CAD build for the part. Positions are in the model's coordinates, mm. Round coordinates to 2 decimals unless told otherwise and drop trailing zeros. Write each loop counter-clockwise with the first axis right and the second up, starting at its lowest first coordinate (ties: lowest second). Pieces come first, ordered by that corner, then holes. Notation, with made-up numbers: (11, 62) -> (62, 62) arc R28 cw to (62, 84) -> close; hole circle Ø11 at (80, 35). An arc over 180 degrees is marked (long way). Put each result on its own line as item: value. Start each with the question number.
1. Saw through at B-B on z = 1.85. List the corners of the cut face in (x, y), and give its area (3 significant figures).
2. Drill centre lines: line 1 (Y direction, x = 54, z = 1.7); line 2 (Y direction, x = -5.5, z = 2); line 3 (X direction, y = 4.5, z = 1.25). Where is each one in solid material? Low to high. Write a range as from..to.
3. Pull direction Y, two halves, no side cores. Call faces 1 (the cylindrical face through (60.49, 12.15, 2.03)), 2 (the cylindrical face through (52.52, 8.61, 1.97)), 3 (the flat face through (-1, 0, 4)): pulls with the +Y half, pulls with the -Y half, needs draft (parallel to the pull), parting line crosses it, or undercut.
4. Flat gauge pins, fed straight in: P1, Ø2.5, axis at x = 54, y = -8, coming from the -Z side; P2, Ø1, axis at y = -6, z = 2.5, coming from the -X side. Where does each tip first touch, or does it go through?
5. Saw through at A-A on x = -13.5. List the corners of the cut face in (y, z).
from build123d import *

# Parameters (mm, degrees)
ESBO_O1_W                = 127
ESBO_O1_H                = 30
ESBO_O1_R                = 3
ESBO_O1_R_2              = 1.6
RESSALTO_EXTRUS_O1_DEPTH = 4
FILETE1_R                = 10


with BuildPart() as part:
    # Esboço1 → Ressalto-extrusão1 (new body)
    with BuildSketch(Plane.XY):
        Rectangle(ESBO_O1_W, ESBO_O1_H)
        with Locations((-13.5, 4)):
            Circle(ESBO_O1_R, mode=Mode.SUBTRACT)
        with Locations((-5.5, 4)):
            Circle(ESBO_O1_R_2, mode=Mode.SUBTRACT)
        with Locations((-21.5, 4)):
            Circle(ESBO_O1_R_2, mode=Mode.SUBTRACT)
        with Locations((-54, 8)):
            Circle(ESBO_O1_R_2, mode=Mode.SUBTRACT)
        with Locations(Location((-54, -8, 0), (0, 0, 180))):
            Circle(ESBO_O1_R_2, mode=Mode.SUBTRACT)
        with Locations((54, -8)):
            Circle(ESBO_O1_R_2, mode=Mode.SUBTRACT)
        with Locations(Location((54, 8, 0), (0, 0, 180))):
            Circle(ESBO_O1_R_2, mode=Mode.SUBTRACT)
    extrude(amount=RESSALTO_EXTRUS_O1_DEPTH)

    # Filete1
    filete1_edges = [part.edges().sort_by_distance(p)[0] for p in [
        (63.5, -15, 2),
        (-63.5, -15, 2),
        (-63.5, 15, 2),
        (63.5, 15, 2),
    ]]
    fillet(filete1_edges, radius=FILETE1_R)


solid = part.part
Return value:
1. outline: (-63.5, -5) arc R10 ccw to (-53.5, -15) -> (53.5, -15) arc R10 ccw to (63.5, -5) -> (63.5, 5) arc R10 ccw to (53.5, 15) -> (-53.5, 15) arc R10 ccw to (-63.5, 5) -> close; hole circle Ø3.2 at (-54, -8); hole circle Ø3.2 at (-54, 8); hole circle Ø3.2 at (-21.5, 4); hole circle Ø6 at (-13.5, 4); hole circle Ø3.2 at (-5.5, 4); hole circle Ø3.2 at (54, -8); hole circle Ø3.2 at (54, 8)
1. area: 3,650 mm^2
2. line 1: y = -14.99..-9.6, -6.4..6.4, 9.6..14.99
2. line 2: y = -15..2.4, 5.6..15
2. line 3: x = -63.5..-23.02, -19.98..-16.46, -10.54..-7.02, -3.98..63.5
3. face 1: pulls with the +Y half
3. face 2: undercut
3. face 3: needs draft
4. P1: passes through
4. P2: stops at x = -63.49
5. outline: (-15, 0) -> (1, 0) -> (1, 4) -> (-15, 4) -> close; (7, 0) -> (15, 0) -> (15, 4) -> (7, 4) -> close
